Input: part model. Units: mm. Frame: model coordinates. Face numbers are marked on the shaded views. Coordinates: 2 decimals unless noted, no trailing zeros. Order: outer loops, then holes, each group sorted by start corner. A loop starts at its lowest first (then second) coordinate and runs counter-clockwise, first axis right, second up. Notation, with made-up numbers: (88.25, 32.5) -> (103.25, 32.5) arc R24 cw to (103.25, 51.5) -> close; hole circle Ø3 at (57, 59.25). An arc over 180 degrees is marked (long way). Write each question's results on one line, items separated by ' | '.
```python
from build123d import *

# Parameters (mm, degrees)
SKETCH2_R           = 16.5
BOSS_EXTRUDE1_DEPTH = 0.5
BOSS_EXTRUDE2_START = 0.5
SKETCH3_R           = 16.5
BOSS_EXTRUDE2_DEPTH = 0.5
SKETCH4_R           = 1
CUT_EXTRUDE1_DEPTH  = 7
SKETCH5_R           = 4
CUT_EXTRUDE2_DEPTH  = 10


with BuildPart() as part:
    # Sketch1 → Revolve1 (revolve)
    with BuildSketch(Plane.XY, mode=Mode.PRIVATE) as revolve1_sk:
        Polygon((0, 6), (0, 0), (13.5, 0), (13.5, 3), (13.5, 6), align=None)
        with BuildLine():
            Line((13.5, 6), (13.5, 3))
            ThreePointArc((13.5, 3), (14.378679656, 5.121320344), (16.5, 6))
            Line((16.5, 6), (13.5, 6))
        make_face()
        with BuildLine():
            Line((13.5, 3), (13.5, 0))
            Line((13.5, 0), (16.5, 0))
            ThreePointArc((16.5, 0), (14.378679656, 0.878679656), (13.5, 3))
        make_face()
    revolve(revolve1_sk.sketch.rotate(Axis((0, 0, 0), (0, 1, 0)), 90), axis=Axis((0, 0, 0), (0, 1, 0)))

    # Sketch2 → Boss-Extrude1 (add)
    with BuildSketch(Plane(origin=(0, 6, 0), x_dir=(1, 0, 0), z_dir=(0, 1, 0))):
        with Locations(Location((0, 0, 0), (0, 0, 270))):
            Circle(SKETCH2_R)
    extrude(amount=BOSS_EXTRUDE1_DEPTH)

    # Sketch3 → Boss-Extrude2 (add)
    with BuildSketch(Plane.XZ.offset(BOSS_EXTRUDE2_START)):
        with Locations(Location((0, 0, 0), (0, 0, 90))):
            Circle(SKETCH3_R)
    extrude(amount=-BOSS_EXTRUDE2_DEPTH)

    # Sketch4 → Cut-Extrude1 (cut)
    with BuildSketch(Plane.XZ.offset(0.5)):
        with Locations(Location((0, 0, 0), (0, 0, 270))):
            Circle(SKETCH4_R)
    extrude(amount=-CUT_EXTRUDE1_DEPTH, mode=Mode.SUBTRACT)

    # Sketch5 → Cut-Extrude2 (cut)
    with BuildSketch(Plane(origin=(0, 6.5, 0), x_dir=(1, 0, 0), z_dir=(0, 1, 0))):
        with Locations(Location((0, 0, 0), (0, 0, 270))):
            Circle(SKETCH5_R)
    extrude(amount=-CUT_EXTRUDE2_DEPTH, mode=Mode.SUBTRACT)


solid = part.part
```
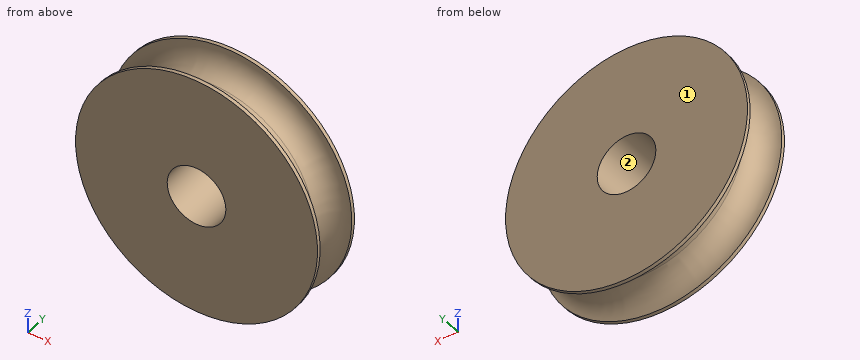
(1) Mould query, pull axis Z, two halves, no side actions, for the marked faces 1 and 2. Classes: +Z half, -Z half, draft (parallel to the pull), parting line (faces both ways), or undercut.
Return value:
face 1: draft | face 2: undercut
(2) Line query: line 1 along Y through (x, z) = (-12.5, 10.5); line 2 along X through (y, z) = (3, 0); line 3 along X through (y, z) = (3.25, 3). Output: solid intervals per line, ascending. Write a range as from..to.
Return value:
line 1: -0.5..0.01, 5.99..6.5 | line 2: -13.5..-4, 4..13.5 | line 3: -13.17..-2.65, 2.65..13.17
(3) Cut plane A-A, the plane z = 0. Return loops of the section in (x, y), plus the area to 3 significant figures.
Return value:
outline: (-16.5, -0.5) -> (-4, -0.5) -> (-4, 6.5) -> (-16.5, 6.5) -> (-16.5, 6) arc R3 cw to (-16.5, 0) -> close; (4, -0.5) -> (16.5, -0.5) -> (16.5, 0) arc R3 cw to (16.5, 6) -> (16.5, 6.5) -> (4, 6.5) -> close | area: 147 mm2
(4) Cut plane B-B, the plane y = 4.75. Return loops of the section in (x, z), plus the area to 3 significant figures.
Return value:
outline: circle Ø28.13 at (0, 0); hole circle Ø8 at (0, 0) | area: 571 mm2
(5) Pin query (flat end, axial travel): P1, Ø1.5, axis at x = -13, y = 5.5, coming from the -Z side; P2, Ø1, axis at x = -8, y = 1, coming from the +Z side. Return the tip coordinate at first contact, or that it passes through.
Return value:
P1: z = -10.84 | P2: z = 12.56
